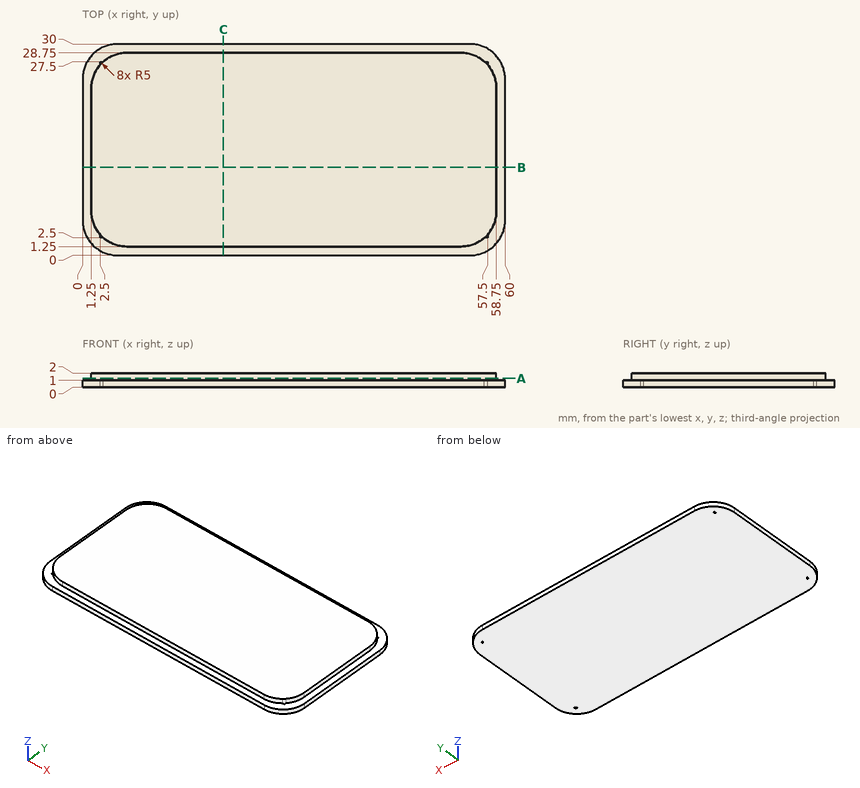
Geometry: see drawing. Coordinates: mm, zero at the bounding-box minimum. Give positions to 0.01 mm unless a question says otherwise; leave off trailing zeros. Loops run counter-clockwise (first coordinate to the right, second up) from the corner with the lowest first, then second, coordinate; pieces in that order, holes last. Notation, with made-up numbers: (-31, 73.25) -> (10, 73.25) arc R23 ccw to (10, 106.25) -> close; hole circle Ø5 at (27, 45). An arc over 180 degrees is marked (long way). Use one line per item in the form item = value.
Item 1: Section query C-C on x = 20. Output: boundary loops of the cut face in (y, z), and give its area (3 significant figures).
A:
outline = (0, 0) -> (30, 0) -> (30, 1) -> (28.75, 1) -> (28.75, 2) -> (1.25, 2) -> (1.25, 1) -> (0, 1) -> close
area = 57.5 mm^2
Item 2: Section query B-B on y = 12.5. Output: boundary loops of the cut face in (x, z).
A:
outline = (0, 0) -> (60, 0) -> (60, 1) -> (58.75, 1) -> (58.75, 2) -> (1.25, 2) -> (1.25, 1) -> (0, 1) -> close
Item 3: Pin query (flat end, axial travel): P1, Ø0.5, axis at x = 57, z = 0.5, coming from the -Y side; P2, Ø0.5, axis at y = 27.5, z = 0.5, coming from the +X side; P3, Ø0.5, axis at y = 27.5, z = 0.5, coming from the -X side. Return the tip coordinate at first contact, or that it passes through.
A:
P1 = 0.32
P2 = 59.47
P3 = 0.53
Item 4: Line query: probe 1 along X at (y, z) = (7, 1.75); probe 2 along Y at (x, z) = (25, 1.2); probe 3 along Y at (x, z) = (57, 0.2). Output: solid intervals per line, ascending.
A:
probe_1 = 1.25 to 58.75
probe_2 = 1.25 to 28.75
probe_3 = 0.42 to 29.58
Item 5: Section query A-A on z = 1.3. Output: boundary loops of the cut face in (x, y), and give its area (3 significant figures).
A:
outline = (1.25, 6.25) arc R5 ccw to (6.25, 1.25) -> (53.75, 1.25) arc R5 ccw to (58.75, 6.25) -> (58.75, 23.75) arc R5 ccw to (53.75, 28.75) -> (6.25, 28.75) arc R5 ccw to (1.25, 23.75) -> close
area = 1,560 mm^2
